Study the drawing (mm; zero at the part's minimum x, y, z) and answer. A direction names the side the tool comes from. Coordinates: 2 decimals unless noted, no trailing zeros. Loops run counter-clockwise (first coordinate to the right, second up) from the corner with the lowest first, then second, coordinate; pieces in that order, holes last. Notation, with made-up numbers: (32, 16) - (76, 16) arc R18 cw to (76, 22) - close; hole circle Ø1 at (0, 52). An arc over 180 degrees is marked (long way). Write each question's results on one line, items separated by ' | '. Start each with the question number.
(1) Find section A-A on x = 29.5. Determine the outline of the cut face in (y, z).
(2) Consider line 1 (Y direction, x = 31, z = 43); line 2 (Y direction, x = 16, z = 18.5); line 3 (Z direction, x = 61.5, y = 28.5). Determine where each line is inside the solid, lowest interval first. Write a range as from..to.
(3) For the marked faces 1 and 2, determine the directions among +Z, -Z, +X, -X, +Y, -Y from which every point of the face is accessible in a straight line to the end or side of a thin tool.
(4) Given pin 1 Ø5 at (x, y) = (22, 70.5) entering from +Z; pin 2 Ø2 at (x, z) = (17, 17) entering from -Y; pin 3 Ø1.3 at (x, z) = (41, 17.5) entering from -Y, each flat-ended and moving along its own axis, determine where each tip first touches the part or whether it passes through.
(5) Find section C-C on y = 100. Determine the outline of the cut face in (x, z), then the cut area to 3 significant figures.
(6) Find section B-B on y = 29.5. Determine the outline of the cut face in (x, z).
(7) Find section D-D on x = 68. Determine the outline of the cut face in (y, z), then the cut area to 3 significant figures.
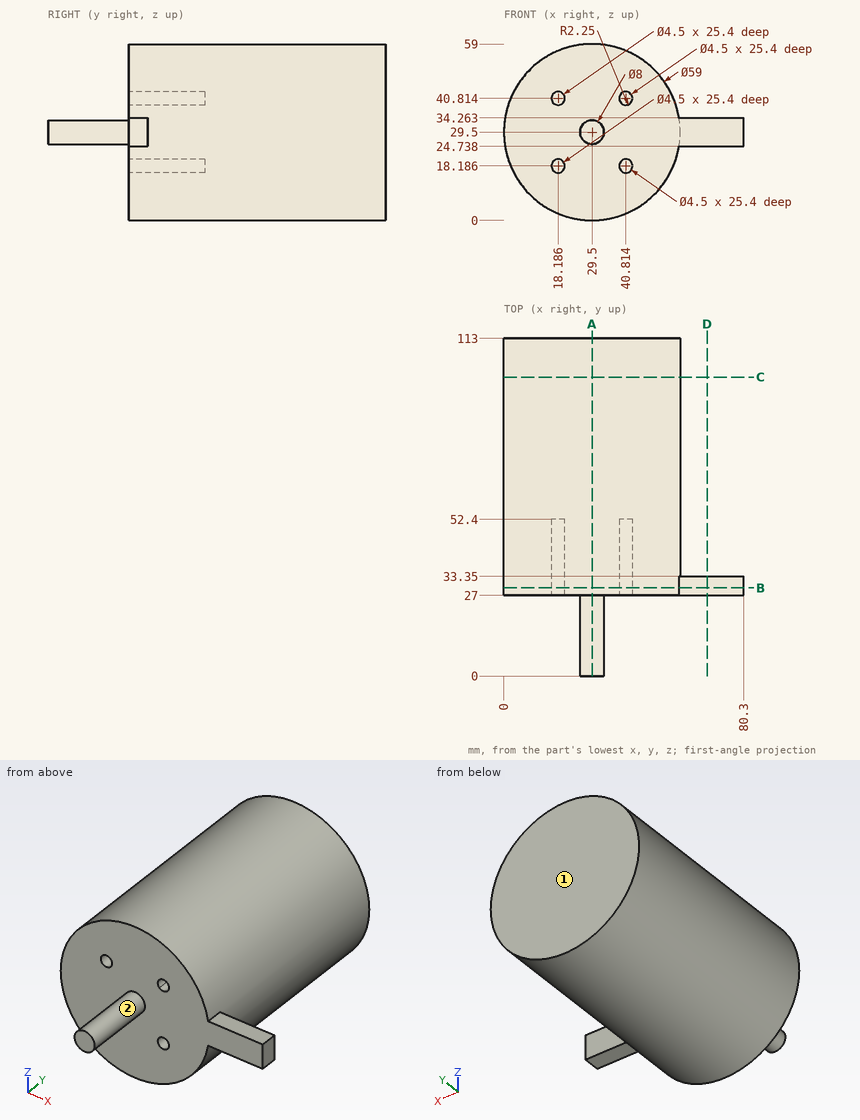
Values:
1) outline: (0, 25.5) - (27, 25.5) - (27, 0) - (113, 0) - (113, 59) - (27, 59) - (27, 33.5) - (0, 33.5) - close
2) line 1: y = 27..113 | line 2: y = 52.4..113 | line 3: z = 24.74..34.26
3) face 1: +Z, -Z, +X, -X, +Y | face 2: -Y
4) pin 1: stops at z = 58.57 | pin 2: stops at y = 27 | pin 3: stops at y = 52.4
5) outline: circle Ø59 at (29.5, 29.5) | area: 2,730 mm²
6) outline: (58.61, 24.74) - (80.3, 24.74) - (80.3, 34.26) - (58.61, 34.26) arc R29.5 ccw (long way) to start; hole circle Ø4.5 at (18.19, 18.19); hole circle Ø4.5 at (18.19, 40.81); hole circle Ø4.5 at (40.81, 18.19); hole circle Ø4.5 at (40.81, 40.81)
7) outline: (27, 24.74) - (33.35, 24.74) - (33.35, 34.26) - (27, 34.26) - close | area: 60.5 mm²
